Could you check a few things on this model? Use its own coordinates, in mm. A direction names the side the tool comes from. Give positions to 0.01 mm unless a question says otherwise; leave off trailing zeros. Order: outer loops, then holes, each group sorted by start corner. A loop starts at its lowest first (then second) coordinate and runs counter-clockwise, first axis right, second up. Notation, with made-up numbers: (53.25, 86) -> (75.25, 86) arc R32 ccw to (75.25, 113) -> close; hole circle Ø10 at (17, -31). An arc over 180 degrees is marked (long way). Write each question's results on one line, items separated by ' | '.
```python
from build123d import *

# Parameters (mm, degrees)
BOSS_EXTRUDE1_DEPTH = 6
FILLET1_R           = 6
FILLET2_R           = 8
CUT_EXTRUDE1_DEPTH  = 17.5
SKETCH5_R           = 2.75
BOSS_EXTRUDE2_DEPTH = 6
CUT_EXTRUDE2_DEPTH  = 104.140903424


with BuildPart() as part:
    # Sketch1 → Boss-Extrude1 (new, symmetric)
    with BuildSketch(Plane(origin=(0, 0, 0), x_dir=(1, 0, 0), z_dir=(0, 1, 0))):
        Polygon((50, 37.5), (50, 22.5), (-50, 22.5), (-50, -22.5), (50, -22.5), (50, -37.5), (-70, -37.5), (-70, 37.5), align=None)
    extrude(amount=BOSS_EXTRUDE1_DEPTH, both=True)

    # Fillet1
    fillet1_edges = [part.edges().sort_by_distance(p)[0] for p in [
        (50, 6, -30),
        (50, -6, -30),
        (50, -6, 30),
        (50, 6, 30),
    ]]
    fillet(fillet1_edges, radius=FILLET1_R - 0.0001)  # a hair under: the kernel refuses the full size

    # Fillet2
    fillet2_edges = [part.edges().sort_by_distance(p)[0] for p in [
        (-50, 0, -22.5),
        (-50, 0, 22.5),
        (-70, 0, 37.5),
        (-70, 0, -37.5),
    ]]
    fillet(fillet2_edges, radius=FILLET2_R)

    # Sketch4 → Cut-Extrude1 (cut, symmetric)
    with BuildSketch(Plane.XY):
        Polygon((-66, 6), (-51, 1.980762114), (-51, 6), align=None)
    extrude(amount=CUT_EXTRUDE1_DEPTH, both=True, mode=Mode.SUBTRACT)

    # Sketch5 → Boss-Extrude2 (add)
    with BuildSketch(Plane(origin=(-2.921161675, -10.901923789, 0), x_dir=(0.9659258262890701, -0.25881904510251424, 0), z_dir=(0.25881904510251424, 0.9659258262890701, 0))):
        with Locations((-58.059575109, 10)):
            Circle(SKETCH5_R)
        with Locations((-58.059575109, -10)):
            Circle(SKETCH5_R)
    extrude(amount=BOSS_EXTRUDE2_DEPTH)

    # Sketch6 → Cut-Extrude2 (cut, through all)
    with BuildSketch(Plane.XY.offset(37.5)):
        with BuildLine():
            Line((42.25, -2.056088519), (42.25, 2.056088519))
            ThreePointArc((42.25, 2.056088519), (44, 2.7), (45.75, 2.056088519))
            Line((45.75, 2.056088519), (45.75, -2.056088519))
            ThreePointArc((45.75, -2.056088519), (44, -2.7), (42.25, -2.056088519))
        make_face()
    extrude(amount=-CUT_EXTRUDE2_DEPTH, mode=Mode.SUBTRACT)


solid = part.part
```
Q1. Suppose I cut it at C-C on z = -5. Please give me the cut outline in (x, y), and give its area (3 significant figures).
Here are the results:
outline: (-70, -6) -> (-50, -6) -> (-50, 6) -> (-51, 6) -> (-51, 1.98) -> (-66, 6) -> (-70, 6) -> close | area: 210 mm²
Q2. For faces 5 (the flat face through (45.75, 0, 30)), 6 (the flat face through (-55, 5, 17.5)), 7 (the flat face through (-25, -6, 24)), 8 (the cylindrical face through (48.196, 4.289, 30.105)), 9 (the flat face through (3, 0, 22.5)), which set-ups out of +Z, -Z, +X, -X, +Y, -Y let a thin tool reach every point of the face, with its end or its side?
Here are the results:
face 5: +Z, -Z | face 6: +Y | face 7: +Z, -Z, +X, -X, -Y | face 8: +Z, -Z, +X, +Y | face 9: +X, +Y, -Y
Q3. I'm going to push flat-ended pins straight in: pin 1 Ø1.2 at (y, z) = (-1, 32) entering from -X; pin 2 Ø3.5 at (y, z) = (3, 2) entering from +X; pin 3 Ø1.5 at (x, y) = (36.5, 7.5) entering from +Z. Where does each tip first touch, or does it pass through?
Here are the results:
pin 1: stops at x = -69.77 | pin 2: stops at x = -50 | pin 3: passes through
Q4. Suppose I cut it at B-B on x = -21.5. Please give me the cut outline in (y, z).
Here are the results:
outline: (-6, -37.5) -> (6, -37.5) -> (6, -22.5) -> (-6, -22.5) -> close; (-6, 22.5) -> (6, 22.5) -> (6, 37.5) -> (-6, 37.5) -> close
Q5. I need wall thicknesses on line 1 along Z through (x, y) = (-16, -4.5); line 2 along Z through (x, y) = (-55, 3.75); line 3 along Y through (x, z) = (-25, 34). Which ranges of each line are inside material? Lowest first, please.
Here are the results:
line 1: z = -37.5 to -22.5, 22.5 to 37.5 | line 2: z = -37.5 to -17.5, 17.5 to 37.5 | line 3: y = -6 to 6
Q6. Thinking about a two-plate mould opening in X: for faces 1 (the flat face through (-70, 0, 0)), 2 (the cylindrical face through (48.289, -4.196, 30.105)), 3 (the flat face through (-12, 6, -26)), 4 (the cylindrical face through (44, 2.7, -29.9)), which applies, +X half, -X half, draft (parallel to the pull), parting line (faces both ways), or undercut?
Here are the results:
face 1: -X half | face 2: +X half | face 3: draft | face 4: undercut
